The listing builds one solid part. Answer for the finished solid, in the listing's coordinates (mm). Face numbers are marked on the shaded views. A direction names the side the tool comes from. Coordinates: 2 decimals unless noted, no trailing zeros. Order: outer loops, then holes, each group sorted by start corner. A loop starts at its lowest first (then second) coordinate and runs counter-clockwise, first axis right, second up. Notation, with made-up numbers: (66.5, 86.25) -> (100.5, 86.25) arc R27 cw to (100.5, 113.25) -> close; hole circle Ø10 at (20.5, 64). An arc over 180 degrees is marked (long way). One line per question, with ' | ' between items.
from build123d import *

# Parameters (mm, degrees)
SKETCH1_W           = 19.812
SKETCH1_H           = 17.272
BOSS_EXTRUDE1_DEPTH = 16.5608
SKETCH2_W           = 10.5156
SKETCH2_H           = 3.2766
BOSS_EXTRUDE2_DEPTH = 1.27
SKETCH3_R           = 8.3439
BOSS_EXTRUDE3_DEPTH = 2.9464
SKETCH4_R           = 7.874
BOSS_EXTRUDE4_DEPTH = 75.184
SKETCH6_R           = 0.508
WIRE_2_DEPTH        = 10.16
LPATTERN1_COUNT     = 7
LPATTERN1_PITCH     = 1.4478
CUT_EXTRUDE1_DEPTH  = 1.778
CIRPATTERN1_COUNT   = 10
SKETCH8_R           = 7.874
SKETCH8_R_2         = 7.366
CUT_EXTRUDE2_DEPTH  = 1.8796
LPATTERN2_COUNT     = 3
LPATTERN2_PITCH     = 4.064


with BuildPart() as part:
    # Sketch1 → Boss-Extrude1 (new body)
    with BuildSketch(Plane.XY):
        Rectangle(SKETCH1_W, SKETCH1_H)
    extrude(amount=BOSS_EXTRUDE1_DEPTH)

    # Sketch2 → Boss-Extrude2 (add)
    with BuildSketch(Plane(origin=(0, 0, 0), x_dir=(-1, 0, 0), z_dir=(0, 0, -1))):
        with Locations((0, 5.7277)):
            Rectangle(SKETCH2_W, SKETCH2_H)
    extrude(amount=BOSS_EXTRUDE2_DEPTH)

    # Sketch3 → Boss-Extrude3 (add)
    with BuildSketch(Plane.XY.offset(16.5608)):
        Circle(SKETCH3_R)
    extrude(amount=BOSS_EXTRUDE3_DEPTH)

    # Sketch4 → Boss-Extrude4 (add)
    with BuildSketch(Plane.XY.offset(19.5072)):
        Circle(SKETCH4_R)
    extrude(amount=BOSS_EXTRUDE4_DEPTH)

    # Sketch5 → Revolve1 (revolve)
    with BuildSketch(Plane(origin=(0, 0, 0), x_dir=(1, 0, 0), z_dir=(0, 1, 0))):
        with BuildLine():
            Line((0, -96.8502), (0, -94.6912))
            Line((0, -94.6912), (7.874, -94.6912))
            ThreePointArc((7.874, -94.6912), (4.082314203, -96.300669445), (0, -96.8502))
        make_face()
    revolve(axis=Axis((0, 0, 96.8502), (0, 0, -1)))

    # Sketch6 → Wire 2 (add)
    with BuildSketch(Plane(origin=(0, 0, -1.27), x_dir=(-1, 0, 0), z_dir=(0, 0, -1))):
        with Locations((-4.3688, 5.7277)):
            Circle(SKETCH6_R)
    wire_2 = extrude(amount=WIRE_2_DEPTH)

    # LPattern1: Wire 2 ×7
    with Locations(*[(-i * LPATTERN1_PITCH, 0, 0) for i in range(1, LPATTERN1_COUNT)]):
        add(wire_2)

    # Sketch7 → Cut-Extrude1 (cut)
    with BuildSketch(Plane(origin=(0, 8.636, 0), x_dir=(1, 0, 0), z_dir=(0, 1, 0))):
        with BuildLine():
            Line((0.5715, -36.6268), (0.5715, -56.4388))
            ThreePointArc((0.5715, -56.4388), (0, -57.0103), (-0.5715, -56.4388))
            Line((-0.5715, -56.4388), (-0.5715, -36.6268))
            ThreePointArc((-0.5715, -36.6268), (0, -36.0553), (0.5715, -36.6268))
        make_face()
        with BuildLine():
            Line((0.5715, -58.7248), (0.5715, -78.5368))
            ThreePointArc((0.5715, -78.5368), (0, -79.1083), (-0.5715, -78.5368))
            Line((-0.5715, -78.5368), (-0.5715, -58.7248))
            ThreePointArc((-0.5715, -58.7248), (0, -58.1533), (0.5715, -58.7248))
        make_face()
    cut_extrude1 = extrude(amount=-CUT_EXTRUDE1_DEPTH, mode=Mode.SUBTRACT)

    # CirPattern1: Cut-Extrude1 ×10 about axis, 4 skipped
    cirpattern1_axis = Axis((0, 0, 0), (0, 0, -1))
    add([cut_extrude1.rotate(cirpattern1_axis, i * 360 / CIRPATTERN1_COUNT) for i in range(1, CIRPATTERN1_COUNT) if i not in (2, 3, 7, 8)], mode=Mode.SUBTRACT)

    # Sketch8 → Cut-Extrude2 (cut)
    with BuildSketch(Plane.XY.offset(82.2452)):
        Circle(SKETCH8_R)
        Circle(SKETCH8_R_2, mode=Mode.SUBTRACT)
    cut_extrude2 = extrude(amount=-CUT_EXTRUDE2_DEPTH, mode=Mode.SUBTRACT)

    # LPattern2: Cut-Extrude2 ×3
    with Locations(*[(0, 0, i * LPATTERN2_PITCH) for i in range(1, LPATTERN2_COUNT)]):
        add(cut_extrude2, mode=Mode.SUBTRACT)


solid = part.part
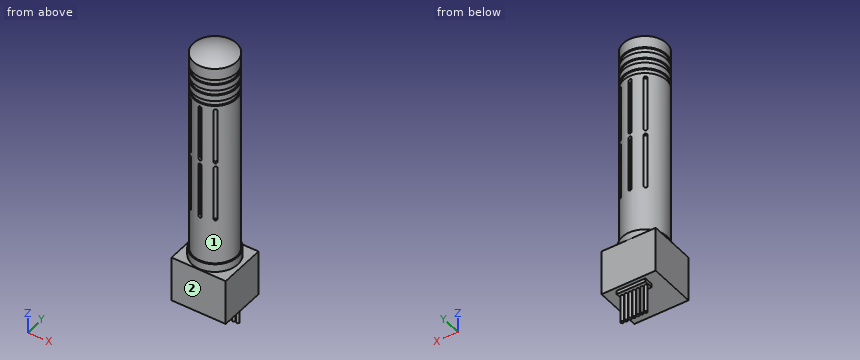
Item 1: Find the intervals of material crossed by L1, parallel to X at y = 7, z = 68.5; L2, parallel to Y at x = -0.5, z = 42.5; L3, parallel to Z at x = -4.75, y = 6.5, in increasing order.
Computed values:
L1: x = -3.61 to -0.57, 0.57 to 3.61 | L2: y = -6.86 to 6.86 | L3: z = -1.27 to 19.51
Item 2: Each of these flat-tipped pins is pushed along its axis until it touches: pin 1 Ø5 at (x, z) = (-2, 65) entering from -Y; pin 2 Ø1 at (x, z) = (1, 32) entering from +Y; pin 3 Ø0.5 at (y, z) = (7.5, 64.5) entering from -X. Where does it stop, or does it pass through?
Computed values:
pin 1: stops at y = -7.85 | pin 2: stops at y = 7.86 | pin 3: stops at x = -3.07
Item 3: For the marked faces 1 and 2, determine the directions among +Z, -Z, +X, -X, +Y, -Y from which every point of the face is accessible in a straight line to the end or side of a thin tool.
Computed values:
face 1: +Z | face 2: +Z, -Z, +X, -X, -Y
Item 4: Section A-A, the plane z = -4.5 is taken. Give the vertices of the cut face in (x, y), plus the area to 3 significant figures.
Computed values:
outline: circle Ø1.02 at (-4.32, 5.73); circle Ø1.02 at (-2.87, 5.73); circle Ø1.02 at (-1.42, 5.73); circle Ø1.02 at (0.03, 5.73); circle Ø1.02 at (1.47, 5.73); circle Ø1.02 at (2.92, 5.73); circle Ø1.02 at (4.37, 5.73) | area: 5.68 mm^2
